Part model, mm, in its own coordinate system. A direction names the side the tool comes from. Round coordinates to 2 decimals unless told otherwise and drop trailing zeros. Loops run counter-clockwise (first coordinate to the right, second up) from the corner with the lowest first, then second, coordinate; pieces in that order, holes last.
from build123d import *

# Parameters (mm, degrees)
F1_DEPTH = 101.6
F3_DEPTH = 95.25
F4_R     = 25.4
F6_DEPTH = 3.81


# Not quite as in the source:
# - a feature names something its author has since deleted; it is built from what else it names


with BuildPart() as f1:
    # F0 (on Top) → F1 (new body)
    with BuildSketch(Plane.XY):
        with BuildLine():
            ThreePointArc((33.8925523579, 0), (-4.2074476421, 84.4010416505), (-42.3074476421, 0))
            Line((-42.3074476421, 0), (33.8925523579, 0))
        make_face()
    extrude(amount=F1_DEPTH)

    # F2 (on face) → F3 (cut)
    with BuildSketch(Plane.XY.offset(101.6)):
        with BuildLine():
            ThreePointArc((33.8925523579, 8.89), (-4.2074476421, 78.3858036913), (-42.3074476421, 8.89))
            Line((-42.3074476421, 8.89), (33.8925523579, 8.89))
        make_face()
    extrude(amount=-F3_DEPTH, mode=Mode.SUBTRACT)

    # F4
    f4_edges = [f1.edges().sort_by_distance(p)[0] for p in [
        (-42.307448, 0, 50.8),
        (33.892552, 0, 50.8),
    ]]
    fillet(f4_edges, radius=F4_R)

    # F5 (on face) → F6 (join)
    with BuildSketch(Plane.XZ):
        Polygon((-28.2470590334, 31.75), (-28.2470590334, 25.4), (-15.5470590334, 25.4), (-15.5470590334, 31.75), (-18.7367527627, 31.75), (-11.6416137586, 49.4294089978), (-4.5464747545, 31.75), (2.5486642496, 49.4294089978), (9.6438032537, 31.75), (7.1321637492, 31.75), (7.1321637492, 25.4), (19.8321637492, 25.4), (19.8321637492, 31.75), (16.0221637492, 31.75), (5.9138143828, 55.0519585676), (12.2638143828, 55.0519585676), (12.2638143828, 61.4019585676), (3.3738143828, 61.4019585676), (-4.2074476421, 43.9254896419), (-11.7887096669, 61.4019585676), (-20.6787096669, 61.4019585676), (-20.6787096669, 55.0519585676), (-14.3287096669, 55.0519585676), (-24.4370590334, 31.75), align=None)
    extrude(amount=F6_DEPTH)


solid = f1.part
1) Tool access for faces 4 (the face through (-1.049, -1.878, 40.466)), 5 (the face through (8, -2, 61.402)), 6 (the face through (19.832, -2, 29)), 7 (the face through (-19.312, -1.878, 43.564)): list every direction of +Z, -Z, +X, -X, +Y, -Y with a clear straight run to the whole face (end or side of a thin tool).
Values:
face 4: -Z, -Y
face 5: +Z, +X, -X, -Y
face 6: +Z, -Z, +X, -Y
face 7: -X, -Y
2) Drop flat-ended pins along their axis: pin 1 Ø1.6 at (x, y) = (-18, -2.5) entering from +Z; pin 2 Ø23 at (x, z) = (-3.5, 63) entering from +Y; pin 3 Ø1 at (y, z) = (36.5, 55.5) entering from +X. Give the stop position or say it passes through.
Values:
pin 1: stops at z = 61.4
pin 2: stops at y = 84.4
pin 3: stops at x = 46.54
3) Slice it at C-C, the plane y = 58. Give the cut face in (x, z), then the cut area to 3 significant figures.
Values:
outline: (-48.76, 0) - (40.35, 0) - (40.35, 101.6) - (33.57, 101.6) - (33.57, 6.35) - (-41.98, 6.35) - (-41.98, 101.6) - (-48.76, 101.6) - close
area: 1,860 mm2
4) Slice it at D-D, the plane z = 8. Give the cut face in (x, y), then the cut area to 3 significant figures.
Values:
outline: (-52.29, 17.2) arc R25.4 ccw to (-28.25, 0) - (19.83, 0) arc R25.4 ccw to (43.87, 17.2) arc R50.8 ccw (long way) to start; hole (-42.31, 8.89) - (33.89, 8.89) arc R45.19 ccw (long way) to start
area: 1,830 mm2
5) Slice it at B-B, the plane x = 26. Give the cut face in (y, z).
Values:
outline: (0.76, 0) - (74.44, 0) - (74.44, 101.6) - (66.81, 101.6) - (66.81, 6.35) - (8.89, 6.35) - (8.89, 101.6) - (0.76, 101.6) - close
6) Slice it at A-A, the plane z = 27. Give the cut face in (x, y).
Values:
outline: (-52.29, 17.2) arc R25.4 ccw to (-28.25, 0) - (-28.25, -3.81) - (-15.55, -3.81) - (-15.55, 0) - (7.13, 0) - (7.13, -3.81) - (19.83, -3.81) - (19.83, 0) arc R25.4 ccw to (43.87, 17.2) arc R50.8 ccw (long way) to start; hole (-42.31, 8.89) - (33.89, 8.89) arc R45.19 ccw (long way) to start
7) Mould opens along Y. For faces 1 (the face through (-2.855, 78.366, 54.642)), 2 (the face through (34.79, 4.87, 51.51)), 3 (the face through (12.264, -2, 58)) say: released by +Y, released by -Y, zero draft, split by the parting line, or undercut.
Values:
face 1: undercut
face 2: released by -Y
face 3: zero draft
8) Wall check: line 1 along X through (y, z) = (33.5, 59); line 2 along Y through (x, z) = (-4.5, 41); line 3 along Z through (x, y) = (15, 56). Give the ranges that are in metal, low to high.
Values:
line 1: x = -55.01 to -49.4, 40.98 to 46.59
line 2: y = -3.81 to 8.89, 78.38 to 84.4
line 3: z = 0 to 6.35
